Design review of the part built by this model. Coordinates are the model's own, in mm. Face numbers are marked on the shaded views. A direction names the side the tool comes from. Round coordinates to 2 decimals unless told otherwise and drop trailing zeros. Loops run counter-clockwise (first coordinate to the right, second up) from the corner with the lowest first, then second, coordinate; pieces in that order, holes last. Notation, with made-up numbers: (51, -23) -> (75, -23) arc R9 cw to (75, -17) -> close; hole circle Ø10 at (-30.5, -17). An arc over 180 degrees is marked (long way). Answer as CSV lines item,"result". Start each with the question number.
```python
from build123d import *

# Parameters (mm, degrees)
F0_W          = 210
F0_H          = 225
F1_DEPTH      = 25
F3_DEPTH      = 95
F5_DEPTH      = 10
F5_DEPTH_BACK = 120
F7_DEPTH      = 10
F7_DEPTH_BACK = 120
F8_W          = 60
F8_H          = 60
F9_DEPTH      = 20
F10_R         = 10
F12_R         = 25.3785837957
F13_DEPTH     = 25.4
F14_R         = 27.9917909544
F15_DEPTH     = 25.4


with BuildPart() as f1:
    # F0 (on Top) → F1 (new body)
    with BuildSketch(Plane.XY):
        Rectangle(F0_W, F0_H)
    extrude(amount=F1_DEPTH)

    # F2 (on face) → F3 (join)
    with BuildSketch(Plane.XY.offset(25)):
        with BuildLine():
            Line((-71, -32.5), (-71, -112.5))
            Line((-71, -112.5), (-56, -112.5))
            Line((-56, -112.5), (-56, -46.4818166789))
            ThreePointArc((-56, -46.4818166789), (7.4888527117, -14.9888527117), (38.9818166789, 48.5))
            Line((38.9818166789, 48.5), (105, 48.5))
            Line((105, 48.5), (105, 63.5))
            Line((105, 63.5), (25, 63.5))
            ThreePointArc((25, 63.5), (-3.1177490061, -4.3822509939), (-71, -32.5))
        make_face()
    extrude(amount=F3_DEPTH)

    # F4 (on face) → F5 (join, two sides)
    with BuildSketch(Plane.XZ.offset(112.5)) as f5_sk:
        with BuildLine():
            ThreePointArc((-56, 83.2576538583), (-34.4526249034, 96.2829175487), (-26, 120))
            ThreePointArc((-26, 120), (-87.2170824513, 149.0473750966), (-71, 83.2576538583))
            Line((-71, 83.2576538583), (-71, 120))
            Line((-71, 120), (-56, 120))
            Line((-56, 120), (-56, 83.2576538583))
        make_face()
        with BuildLine():
            Line((-71, 120), (-71, 83.2576538583))
            ThreePointArc((-71, 83.2576538583), (-63.5, 82.5), (-56, 83.2576538583))
            Line((-56, 83.2576538583), (-56, 120))
            Line((-56, 120), (-71, 120))
        make_face()
    extrude(amount=F5_DEPTH)
    extrude(f5_sk.sketch, amount=-F5_DEPTH_BACK)

    # F6 (on face) → F7 (join, two sides)
    with BuildSketch(Plane.YZ.offset(105)) as f7_sk:
        with BuildLine():
            Line((48.5, 120), (48.5, 83.2576538583))
            ThreePointArc((48.5, 83.2576538583), (56, 82.5), (63.5, 83.2576538583))
            Line((63.5, 83.2576538583), (63.5, 120))
            Line((63.5, 120), (48.5, 120))
        make_face()
        with BuildLine():
            ThreePointArc((63.5, 83.2576538583), (85.0473750966, 96.2829175487), (93.5, 120))
            ThreePointArc((93.5, 120), (32.2829175487, 149.0473750966), (48.5, 83.2576538583))
            Line((48.5, 83.2576538583), (48.5, 120))
            Line((48.5, 120), (63.5, 120))
            Line((63.5, 120), (63.5, 83.2576538583))
        make_face()
    extrude(amount=F7_DEPTH)
    extrude(f7_sk.sketch, amount=-F7_DEPTH_BACK)

    # F8 (on face) → F9 (join)
    with BuildSketch(Plane.XY.offset(25)):
        with Locations((75, -82.5)):
            Rectangle(F8_W, F8_H)
    extrude(amount=F9_DEPTH)

    # F10
    f10_edges = [f1.edges().sort_by_distance(p)[0] for p in [
        (45, -52.5, 35),
    ]]
    fillet(f10_edges, radius=F10_R)

    # F12 (on face) → F13 (cut)
    with BuildSketch(Plane.XZ.offset(122.5)):
        with Locations((-64.7613108158, 119.6997389197)):
            Circle(F12_R)
    extrude(amount=-F13_DEPTH, mode=Mode.SUBTRACT)

    # F14 (on face) → F15 (cut)
    with BuildSketch(Plane.YZ.offset(115)):
        with Locations((56, 120)):
            Circle(F14_R)
    extrude(amount=-F15_DEPTH, mode=Mode.SUBTRACT)


solid = f1.part
```
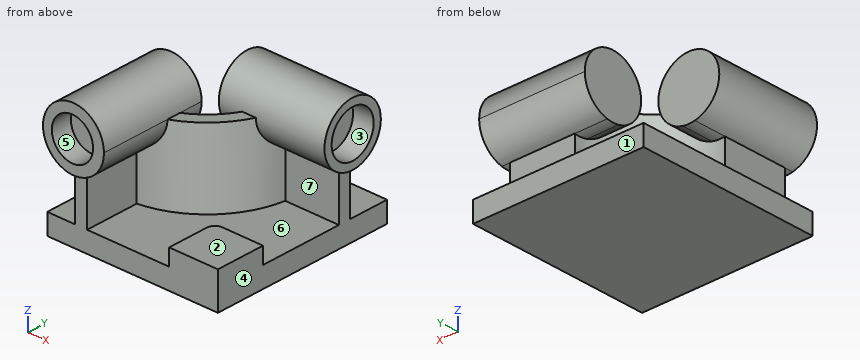
Q1. Add section C-C, the plane z = 58. Give the boundary of the cut face in (x, y), and give its area (3 significant figures).
Q2. To check wall thickness, follow probe 1 along Z at (x, y) = (95, 56); probe 2 along Z at (x, y) = (75.5, -64); probe 3 along Y at (x, z) = (43, 43.5). State the ranges of each line that lie inside material, in increasing order. Write a range as from..to.
Q3. Machinability: for the marked faces 4, 5, 6 and 7, which of the approach directions +Z, -Z, +X, -X, +Y, -Y give a long, thin tool a straight path to every point of the face, cutting with its end or side? Answer none if there is none.
Q4. Add section A-A, the plane x = 6. Give the boundary of the cut face in (y, z).
Q5. Mouldability with a two-part tool opening along Z and no side actions: class the marked faces 1, 2 and 3 as pulls with the +Z half, pulls with the -Z half, needs draft (parallel to the pull), parting line crosses it, or undercut.
Q6. Add section B-B, the plane y = 74. Give the boundary of the cut face in (x, z), and give its area (3 significant figures).
Q7. For pin 1 Ø10 at (y, z) = (-86, 33) entering from -X; pin 2 Ø4 at (y, z) = (-20.5, 27.5) entering from +X; pin 3 Ø25 at (x, z) = (-26.5, 48) entering from -Y, all flat-tipped, find the tip position at first contact; note any pin that passes through.
Q8. Add section D-D, the plane x = 98. Give the boundary of the cut face in (y, z), and give its area (3 significant figures).
Worked answers:
1,outline,"(-71, -112.5) -> (-56, -112.5) -> (-56, -46.48) arc R111 ccw to (38.98, 48.5) -> (105, 48.5) -> (105, 63.5) -> (25, 63.5) arc R96 cw to (-71, -32.5) -> close"
1,area,"4,400 mm^2"
2,probe 1,"z = 0..92.01, 147.99..157.5"
2,probe 2,"z = 0..45"
2,probe 3,"y = 48.5..63.5"
3,face 4,"-Z, +X, +Y, -Y"
3,face 5,"-Y"
3,face 6,"none"
3,face 7,"+X"
4,outline,"(-112.5, 0) -> (112.5, 0) -> (112.5, 25) -> (6.17, 25) -> (6.17, 120) -> (-16.45, 120) -> (-16.45, 25) -> (-112.5, 25) -> close; circle Ø75 at (56, 120)"
5,face 1,"needs draft"
5,face 2,"pulls with the +Z half"
5,face 3,"undercut"
6,outline,"(-105, 0) -> (105, 0) -> (105, 25) -> (-105, 25) -> close; (-15, 87.1) -> (115, 87.1) -> (115, 98.56) -> (89.6, 98.56) -> (89.6, 141.44) -> (115, 141.44) -> (115, 152.9) -> (-15, 152.9) -> close"
6,area,"12,700 mm^2"
7,pin 1,"stops at x = -71"
7,pin 2,"stops at x = 3.81"
7,pin 3,"stops at y = -42.79"
8,outline,"(-112.5, 0) -> (112.5, 0) -> (112.5, 25) -> (63.5, 25) -> (63.5, 83.26) arc R37.5 ccw (long way) to (48.5, 83.26) -> (48.5, 25) -> (-52.5, 25) -> (-52.5, 45) -> (-112.5, 45) -> close; hole circle Ø55.98 at (56, 120)"
8,area,"9,650 mm^2"
